from build123d import *

# Parameters (mm, degrees)
SKETCH_1_R          = 2
EXTRUDE_1_DEPTH     = 8
EXTRUDE_2_DEPTH     = 39
EXTRUDE_3_DEPTH     = 55
SKETCH_4_R          = 4.5
CUT_EXTRUDE_1_DEPTH = 55
FILLET_1_R          = 1
CHAMFER_1_SIZE      = 0.2


with BuildPart() as part:
    # 草图1 → 凸台-拉伸1 (new body)
    with BuildSketch(Plane(origin=(0, 0, 0), x_dir=(0, 0, -1), z_dir=(1, 0, 0))):
        with BuildLine():
            Line((0, 4.5), (4.5, 4.5))
            Line((4.5, 4.5), (4.5, -4.5))
            Line((4.5, -4.5), (-1.5, -4.5))
            ThreePointArc((-1.5, -4.5), (-3.621320344, -3.621320344), (-4.5, -1.5))
            Line((-4.5, -1.5), (-4.5, 1.5))
            ThreePointArc((-4.5, 1.5), (-3.621320344, 3.621320344), (-1.5, 4.5))
            Line((-1.5, 4.5), (0, 4.5))
        make_face()
        Circle(SKETCH_1_R, mode=Mode.SUBTRACT)
    extrude(amount=EXTRUDE_1_DEPTH)

    # 草图2 → 凸台-拉伸2 (add)
    with BuildSketch(Plane(origin=(0, 0, -4.5), x_dir=(-1, 0, 0), z_dir=(0, 0, -1))):
        Polygon((-4, 10), (3.5, 10), (3.5, -10), (-11.5, -10), (-11.5, 10), align=None)
    extrude(amount=EXTRUDE_2_DEPTH)

    # 草图3 → 凸台-拉伸3 (add)
    with BuildSketch(Plane(origin=(0, 0, -43.5), x_dir=(-1, 0, 0), z_dir=(0, 0, -1))):
        with BuildLine():
            Line((2.5, 6.224949799), (2.5, -6.224949799))
            ThreePointArc((2.5, -6.224949799), (-4, -9), (-10.5, -6.224949799))
            Line((-10.5, -6.224949799), (-10.5, 6.224949799))
            ThreePointArc((-10.5, 6.224949799), (-4, 9), (2.5, 6.224949799))
        make_face()
    extrude(amount=EXTRUDE_3_DEPTH)

    # 草图4 → 切除-拉伸1 (cut)
    with BuildSketch(Plane(origin=(0, 0, -98.5), x_dir=(-1, 0, 0), z_dir=(0, 0, -1))):
        with Locations(Location((-4, 0, 0), (0, 0, 90))):
            Circle(SKETCH_4_R)
    extrude(amount=-CUT_EXTRUDE_1_DEPTH, mode=Mode.SUBTRACT)

    # 圆角1
    fillet_1_edges = [part.edges().sort_by_distance(p)[0] for p in [
        (4, -10, -4.5),
        (4, 10, -4.5),
        (4, 10, -43.5),
        (4, -10, -43.5),
    ]]
    fillet(fillet_1_edges, radius=FILLET_1_R - 0.0001)  # a hair under: the kernel refuses the full size

    # 倒角1
    chamfer_1_edges = [part.edges().sort_by_distance(p)[0] for p in [
        (-3.5, -10, -24),
        (11.5, -10, -24),
        (-3.5, 0, -4.5),
        (-3.5, 10, -24),
        (-3.5, 0, -43.5),
        (-3.5, 9.707136071, -4.792863929),
        (-3.5, 9.707136071, -43.207136071),
        (-3.5, -9.707136071, -43.207136071),
        (-3.5, -9.707136071, -4.792863929),
        (11.5, 0, -4.5),
        (11.5, 0, -43.5),
        (11.5, 10, -24),
        (11.5, 9.707136071, -4.792863929),
        (11.5, 9.707136071, -43.207136071),
        (11.5, -9.707136071, -43.207136071),
        (11.5, -9.707136071, -4.792863929),
    ]]
    chamfer(chamfer_1_edges, length=CHAMFER_1_SIZE)


solid = part.part
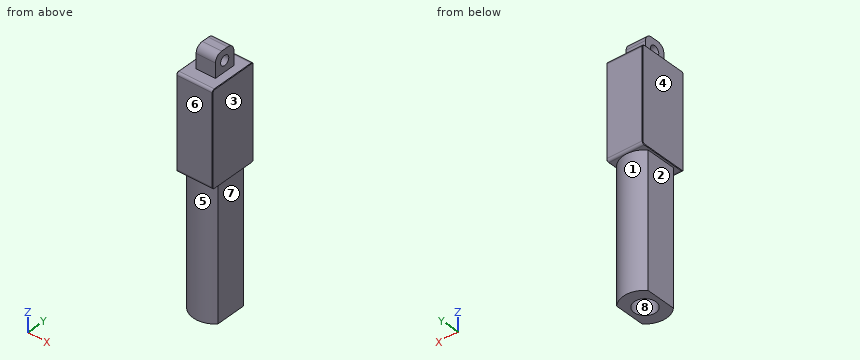
Build history of the part. All positions in model axes, mm. Face numbers are marked on the shaded views. A direction names the side the tool comes from. Round coordinates to 2 decimals unless told otherwise and drop trailing zeros. Write each loop counter-clockwise with the first axis right and the second up, starting at its lowest first coordinate (ties: lowest second). Pieces come first, ordered by that corner, then holes. Notation, with made-up numbers: M 2.5,26 L 30.5,26 A25 ccw 30.5,62 Z; hole C 10,86.25 d3. An arc over 180 degrees is marked long. Answer in a Markdown table with one row per item.
1. Mould opens along Y. For the marked faces 6, 7 and 8 say: +Y half, -Y half, draft (parallel to the pull), parting line (faces both ways), or undercut.
Geometry check:
| item | result |
|---|---|
| face 6 | -Y half |
| face 7 | draft |
| face 8 | undercut |
2. Which spindle directions (+Z, -Z, +X, -X, +Y, -Y) get a long thin tool onto all of the face, cutting with end or side? Do the marked faces 1, 2, 3, 4 and 5. Say none if no direction does.
Geometry check:
| item | result |
|---|---|
| face 1 | -Z, +Y |
| face 2 | -Z, -X, +Y, -Y |
| face 3 | +Z, -Z, +X, +Y, -Y |
| face 4 | +Z, -Z, -X, +Y, -Y |
| face 5 | -Z, -Y |
3. Flat gauge pins, fed straight in: P1, Ø4.5, axis at y = 1, z = -1.5, coming from the -X side; P2, Ø3, axis at x = 4.5, z = -1.5, coming from the -Y side; P3, Ø3, axis at y = -6, z = -71.5, coming from the -X side; P4, Ø3.5, axis at y = 0, z = 0, coming from the -X side. Where does each tip first touch, or does it go through?
Geometry check:
| item | result |
|---|---|
| P1 | x = 0 |
| P2 | y = -4.5 |
| P3 | x = -2.5 |
| P4 | through |
4. Probe L1, parallel to X at y = 0, z = -74.5; L2, parallel to Y at x = 3.75, z = 0; L3, parallel to Z at x = 5, y = -9. List the from-to ranges inside material, lowest first. Write a range as [from, to].
Geometry check:
| item | result |
|---|---|
| L1 | [-2.5, -0.5], [8.5, 10.5] |
| L2 | [-4.5, -2], [2, 4.5] |
| L3 | [-43.5, -4.5] |
5. Saw through at B-B (y = 0). List the corners of the cut face in (x, z), and give its area (3 significant figures).
Geometry check:
| item | result |
|---|---|
| outline | M -3.5,-43.3 L -3.3,-43.5 L -2.5,-43.5 L -2.5,-98.5 L -0.5,-98.5 L -0.5,-43.5 L 8.5,-43.5 L 8.5,-98.5 L 10.5,-98.5 L 10.5,-43.5 L 11.3,-43.5 L 11.5,-43.3 L 11.5,-4.7 L 11.3,-4.5 L 8,-4.5 L 8,-2 L 0,-2 L 0,-4.5 L -3.3,-4.5 L -3.5,-4.7 Z; M 0,2 L 8,2 L 8,4.5 L 0,4.5 Z |
| area | 845 mm2 |
6. Saw through at C-C (z = -75). List the corners of the cut face in (x, y), and give its area (3 significant figures).
Geometry check:
| item | result |
|---|---|
| outline | M -2.5,-6.22 A9 ccw 10.5,-6.22 L 10.5,6.22 A9 ccw -2.5,6.22 Z; hole C 4,0 d9 |
| area | 148 mm2 |
